Verification items for the finished model (mm, model axes). A direction names the side the tool comes from. Round coordinates to 2 decimals unless told otherwise and drop trailing zeros. Loops run counter-clockwise (first coordinate to the right, second up) from the corner with the lowest first, then second, coordinate; pieces in that order, holes last. Notation, with made-up numbers: M -39,-14.75 L 9,-14.75 A16 ccw 9,5.25 Z; hole C 22,44.5 d1. An arc over 180 degrees is marked long. Answer as CSV lines item,"result".
```python
from build123d import *

# Parameters (mm, degrees)
SKETCH1_R           = 1.05
BOSS_EXTRUDE1_DEPTH = 2.85
FILLET2_R           = 1
FILLET1_R           = 1


with BuildPart() as part:
    # Sketch1 → Boss-Extrude1 (new body)
    with BuildSketch(Plane.XY):
        with BuildLine():
            Line((2.236067977, 2), (8.5, 3.5))
            Line((8.5, 3.5), (8.5, 6))
            ThreePointArc((8.5, 6), (10.130733614, 7.494292047), (11.47721163, 5.739527733))
            Line((11.47721163, 5.739527733), (10.729668505, 1.5))
            Line((10.729668505, 1.5), (0, -2))
            Line((0, -2), (-10.729668505, 1.5))
            Line((-10.729668505, 1.5), (-11.47721163, 5.739527733))
            ThreePointArc((-11.47721163, 5.739527733), (-10.130733614, 7.494292047), (-8.5, 6))
            Line((-8.5, 6), (-8.5, 3.5))
            Line((-8.5, 3.5), (-2.236067977, 2))
            ThreePointArc((-2.236067977, 2), (0, 3), (2.236067977, 2))
        make_face()
        Circle(SKETCH1_R, mode=Mode.SUBTRACT)
    extrude(amount=BOSS_EXTRUDE1_DEPTH)

    # Fillet2
    fillet2_edges = [part.edges().sort_by_distance(p)[0] for p in [
        (8.5, 3.5, 1.425),
        (-8.5, 3.5, 1.425),
    ]]
    fillet(fillet2_edges, radius=FILLET2_R)

    # Fillet1
    fillet1_edges = [part.edges().sort_by_distance(p)[0] for p in [
        (8.5, 5.144403083, 0),
        (10.130733614, 7.494292047, 0),
        (11.103440067, 3.619763867, 0),
        (-11.103440067, 3.619763867, 0),
        (-10.130733614, 7.494292047, 0),
        (-10.130733614, 7.494292047, 2.85),
        (-4.984475025, 2.658150592, 0),
        (-11.103440067, 3.619763867, 2.85),
        (11.103440067, 3.619763867, 2.85),
        (10.130733614, 7.494292047, 2.85),
        (8.5, 5.144403083, 2.85),
        (-8.5, 5.144403083, 0),
        (-8.5, 5.144403083, 2.85),
        (4.984475025, 2.658150592, 0),
        (4.984475025, 2.658150592, 2.85),
        (-8.285137591, 3.669484793, 0),
        (-8.285137591, 3.669484793, 2.85),
        (8.285137591, 3.669484793, 0),
        (8.285137591, 3.669484793, 2.85),
        (-4.984475025, 2.658150592, 2.85),
    ]]
    fillet(fillet1_edges, radius=FILLET1_R)


solid = part.part
```
1) Section check B-B (y = 0.25). Record the cut outline in (x, z), plus the area to 3 significant figures.
Here are the results:
outline,"M -6.9,0 L -1.02,0 L -1.02,2.85 L -6.9,2.85 Z; M 1.02,0 L 6.9,0 L 6.9,2.85 L 1.02,2.85 Z"
area,"33.5 mm^2"
2) Section check A-A (z = 1.3). Record the cut outline in (x, y).
Here are the results:
outline,"M -11.48,5.74 L -10.73,1.5 L 0,-2 L 10.73,1.5 L 11.48,5.74 A1.5 ccw long 8.5,6 L 8.5,4.29 A1 cw 7.73,3.32 L 2.24,2 A3 ccw -2.24,2 L -7.73,3.32 A1 cw -8.5,4.29 L -8.5,6 A1.5 ccw long Z; hole C 0,0 d2.1"
3) Material ranges on probe 1 along Y at (x, z) = (0, 0.6); probe 2 along X at (y, z) = (5.5, 0.7); probe 3 along X at (y, z) = (6.5, 0.5), recorded low to high.
Here are the results:
probe 1,"y = -2 to -1.05, 1.05 to 3"
probe 2,"x = -11.39 to -8.55, 8.55 to 11.39"
probe 3,"x = -11.27 to -8.73, 8.73 to 11.27"
4) Go/stop test with flat-tipped pins: pin 1 (1 mm diameter, centred on x = 5, y = 3, fed in from -Z); pin 2 (0.7 mm diameter, centred on y = 5, z = 1.5, fed in from -X). Record where each tip stops, or that it passes through.
Here are the results:
pin 1,"stops at z = 0.44"
pin 2,"stops at x = -11.41"
5) Draft check along X on faces 1 (the flat face through (0, 1.3, 2.85)), 2 (the cylindrical face through (10.76, 3.38, 0.29)), 3 (the flat face through (-11.1, 3.6, 1.4)), 4 (the cylindrical face through (8.801, 5.156, 2.565)). Enter one of: +X half, -X half, draft (parallel to the pull), parting line (faces both ways), or undercut.
Here are the results:
face 1,"draft"
face 2,"+X half"
face 3,"-X half"
face 4,"undercut"
6) Set-up check for faces 5 (the cylindrical face through (-5.02, 2.36, 0.29)), 6 (the cylindrical face through (-8.28, 3.66, 1.43)), 7 (the cylindrical face through (-5.02, 2.36, 2.56)), 8 (the cylindrical face through (-10.77, 3.44, 0.29)): record each of +Z, -Z, +X, -X, +Y, -Y from which the full face is reachable in a straight line by a thin tool's end or side.
Here are the results:
face 5,"-Z, +Y"
face 6,"+Z, -Z, +Y"
face 7,"+Z, +Y"
face 8,"-Z, -X, -Y"
